from build123d import *

# Parameters (mm, degrees)
F1_DEPTH     = 40.894
F2_T1_DEPTH  = 66.294
F2_T6_DEPTH  = 41.888453839
F2_T11_DEPTH = 41.888453839


# Not quite as in the source:
# - a fillet or chamfer that OpenCascade refuses, or shapes differently, is made with other operations: its cross-section is extruded or revolved along the edge and cut away or added


with BuildPart() as f1:
    # F0 (on Front) → F1 (new body)
    with BuildSketch(Plane.XZ):
        Polygon((-44.7658635676, 39.5274721086), (-44.7658635676, -35.146754235), (64.7440105677, -35.146754235), (64.7440105677, 39.5274721086), (30.9880006403, 39.5274721086), (30.9880006403, 50.7696404397), (5.5880006403, 50.7696404397), (5.5880006403, 39.5274721086), (-2.774850931, 39.5274721086), (-2.774850931, 49.2475219071), (-19.26330477, 49.2475219071), (-19.26330477, 39.5274721086), align=None)
    extrude(amount=F1_DEPTH)

    # F2: fillet of radius 5.08 on 4 edges, made by hand

    # F2_s2 → F2_t1 (cut)
    with BuildSketch(Plane.XZ.offset(-12.7)):
        with BuildLine():
            add(Edge.make_bspline(
                [(-2.774850931, 44.1675219071), (-2.774850931, 49.2475219071), (-7.854850931, 49.2475219071)],
                knots=[0, 0, 0, 1, 1, 1], degree=2, weights=[1, 1, 1]))
            Line((-7.854850931, 49.2475219071), (-2.774850931, 49.2475219071))
            Line((-2.774850931, 49.2475219071), (-2.774850931, 44.1675219071))
        make_face()
        with BuildLine():
            add(Edge.make_bspline(
                [(-14.18330477, 49.2475219071), (-19.26330477, 49.2475219071), (-19.26330477, 44.1675219071)],
                knots=[0, 0, 0, 1, 1, 1], degree=2, weights=[1, 1, 1]))
            Line((-19.26330477, 44.1675219071), (-19.26330477, 49.2475219071))
            Line((-19.26330477, 49.2475219071), (-14.18330477, 49.2475219071))
        make_face()
    extrude(amount=F2_T1_DEPTH, mode=Mode.SUBTRACT)


with BuildPart() as f2_tool4:
    # F2_s5 → F2_t6 (new body)
    with BuildSketch(Plane.YZ.offset(9.925149069)):
        with BuildLine():
            add(Edge.make_bspline(
                [(-5.08, 49.2475219071), (0, 49.2475219071), (0, 44.1675219071)],
                knots=[0, 0, 0, 1, 1, 1], degree=2, weights=[1, 1, 1]))
            Line((0, 44.1675219071), (0, 49.2475219071))
            Line((0, 49.2475219071), (-5.08, 49.2475219071))
        make_face()
    extrude(amount=-F2_T6_DEPTH)

    split(bisect_by=Plane.YZ.offset(5.5880006403), keep=Keep.BOTTOM)


with BuildPart() as f1_1:
    add(f1.part)

    # F2_t3: cut F2_tool4
    add(f2_tool4.part, mode=Mode.SUBTRACT)


with BuildPart() as f2_tool9:
    # F2_s10 → F2_t11 (new body)
    with BuildSketch(Plane.YZ.offset(9.925149069)):
        with BuildLine():
            add(Edge.make_bspline(
                [(-35.814, 49.2475219071), (-40.894, 49.2475219071), (-40.894, 44.1675219071)],
                knots=[0, 0, 0, 1, 1, 1], degree=2, weights=[1, 1, 1]))
            Line((-40.894, 44.1675219071), (-40.894, 49.2475219071))
            Line((-40.894, 49.2475219071), (-35.814, 49.2475219071))
        make_face()
    extrude(amount=-F2_T11_DEPTH)

    split(bisect_by=Plane.YZ.offset(5.5880006403), keep=Keep.BOTTOM)


with BuildPart() as f1_2:
    add(f1_1.part)

    # F2_t8: cut F2_tool9
    add(f2_tool9.part, mode=Mode.SUBTRACT)


solid = f1_2.part
Read the model definition and answer for the solid it produces. Units are mm, in the model's axes. A direction names the side the tool comes from. Give positions to 0.01 mm unless a question says otherwise; leave off trailing zeros. Write each loop counter-clockwise with the first axis right and the second up, starting at its lowest first coordinate (ties: lowest second). Pieces come first, ordered by that corner, then holes. Notation, with made-up numbers: (77.5, -28.5) - (127.5, -28.5) arc R25 cw to (127.5, 7.5) - close; hole circle Ø10 at (8, -33). An arc over 180 degrees is marked (long way). Use CSV: the item, a comma, the result in double quotes. Start each with the question number.
(1) Find section A-A (z = 42). Give the vertices of the cut face in (x, y).
(2) Determine the mould class of faces 1 (the flat face through (1, -20, 39.527)), 2 (the flat face through (18, -20, 50.77)), 3 (the flat face through (-44.766, -20, 3)) for opening direction X: +X half, -X half, draft (parallel to the pull), parting line (faces both ways), or undercut.
(3) Find section B-B (x = -25). Give the vertices of the cut face in (y, z).
(4) For faces 4 (the flat face through (5.588, -20, 45)), 5 (the flat face through (-32, -20, 39.527)), 6 (the flat face through (48, -20, 39.527)), 7 (the flat face through (64.744, -20, 2)), determine the directions among +Z, -Z, +X, -X, +Y, -Y from which every point of the face is accessible in a straight line to the end or side of a thin tool.
(5) Consider line 1 along Z through (x, y) = (43.5, -22.5); line 2 along X through (y, z) = (-13, 45.5); line 3 along Z through (x, y) = (-16.5, -26). Determine where each line is inside the solid, lowest interval first.
(6) Given P1, Ø2.5, axis at x = -0.5, y = -22.5, coming from the +Z side; P2, Ø3, axis at x = -10.5, y = -21.5, coming from the +Z side; P3, Ø9, axis at y = -26.5, z = 47, coming from the -X side, each flat-ended and moving along its own axis, determine where each tip first touches the part or whether it passes through.
Findings below:
1,outline,"(-19.26, -40.89) - (-2.77, -40.89) - (-2.77, 0) - (-19.26, 0) - close; (5.59, -40.89) - (30.99, -40.89) - (30.99, 0) - (5.59, 0) - close"
2,face 1,"undercut"
2,face 2,"draft"
2,face 3,"-X half"
3,outline,"(-40.89, -35.15) - (0, -35.15) - (0, 39.53) - (-40.89, 39.53) - close"
4,face 4,"+Z, +Y, -Y"
4,face 5,"+Z, -X, +Y, -Y"
4,face 6,"+Z, +X, +Y, -Y"
4,face 7,"+Z, -Z, +X, +Y, -Y"
5,line 1,"-35.15 to 39.53"
5,line 2,"-19.16 to -2.88, 5.59 to 30.99"
5,line 3,"-35.15 to 48.9"
6,P1,"z = 39.53"
6,P2,"z = 49.25"
6,P3,"x = -19.26"
